Input: part model. Units: mm. Frame: model coordinates. Face numbers are marked on the shaded views. Coordinates: 2 decimals unless noted, no trailing zeros. Write each loop counter-clockwise with the first axis right and the second up, starting at its lowest first coordinate (ties: lowest second). Pieces come first, ordered by that corner, then holes.
1) Section query D-D (x = 15.5). Output: boundary loops of the cut face in (y, z).
2) Section query C-C (y = 4). State how many separate pieces and enclosed holes the cut face has, then the cut area to 3 significant figures.
3) Draft query along Y for the marked faces 1 and 2. Return one class per face: pulls with the +Y half, pulls with the -Y half, needs draft (parallel to the pull), parting line crosses it, or undercut.
4) Section query A-A (x = -4.85). Output: boundary loops of the cut face in (y, z), then the cut area to 4 significant figures.
5) Section query B-B (z = -15.5). Output: boundary loops of the cut face in (x, y), then the cut area to 4 significant figures.
6) Pin query (flat end, axial travel): pin 1 Ø4.5 at (x, z) = (15.15, -28.65) entering from -Y; pin 2 Ø3.5 at (x, z) = (-15.5, 15.5) entering from +Y. Return the tip coordinate at first contact, or that it passes through.
7) Line query: L1, parallel to Z at x = -15.5, y = 2.8; L2, parallel to X at y = 2.55, z = 28.65; L3, parallel to X at y = 2, z = 15.5. Output: solid intervals per line, ascending.
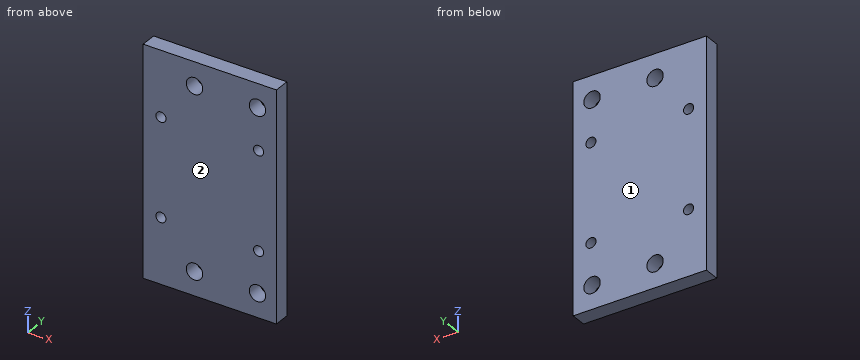
from build123d import *

# Parameters (mm, degrees)
SKETCH2_W           = 42.3
SKETCH2_H           = 42.3
SKETCH2_R           = 1.6
SKETCH2_H_2         = 15
SKETCH2_R_2         = 2.6
BOSS_EXTRUDE1_DEPTH = 5


with BuildPart() as part:
    # Sketch2 → Boss-Extrude1 (new body)
    with BuildSketch(Plane(origin=(0, 0, 0), x_dir=(1, 0, 0), z_dir=(0, 1, 0))):
        Rectangle(SKETCH2_W, SKETCH2_H)
        with Locations((-15.5, -15.5)):
            Circle(SKETCH2_R, mode=Mode.SUBTRACT)
        with Locations((15.5, 15.5)):
            Circle(SKETCH2_R, mode=Mode.SUBTRACT)
        with Locations((15.5, -15.5)):
            Circle(SKETCH2_R, mode=Mode.SUBTRACT)
        with Locations((-15.5, 15.5)):
            Circle(SKETCH2_R, mode=Mode.SUBTRACT)
        with Locations((0, -28.65)):
            Rectangle(SKETCH2_W, SKETCH2_H_2)
        with Locations((15.15, -28.65)):
            Circle(SKETCH2_R_2, mode=Mode.SUBTRACT)
        with Locations((-4.85, -28.65)):
            Circle(SKETCH2_R_2, mode=Mode.SUBTRACT)
        with Locations((0, 28.65)):
            Rectangle(SKETCH2_W, SKETCH2_H_2)
        with Locations((15.15, 28.65)):
            Circle(SKETCH2_R_2, mode=Mode.SUBTRACT)
        with Locations((-4.85, 28.65)):
            Circle(SKETCH2_R_2, mode=Mode.SUBTRACT)
    extrude(amount=BOSS_EXTRUDE1_DEPTH)


solid = part.part
Answer:
1. outline: (0, -36.15) - (5, -36.15) - (5, -31.23) - (0, -31.23) - close; (0, -26.07) - (5, -26.07) - (5, -17.1) - (0, -17.1) - close; (0, -13.9) - (5, -13.9) - (5, 13.9) - (0, 13.9) - close; (0, 17.1) - (5, 17.1) - (5, 26.07) - (0, 26.07) - close; (0, 31.23) - (5, 31.23) - (5, 36.15) - (0, 36.15) - close
2. separate pieces: 1
2. enclosed holes: 8
2. area: 2,940 mm2
3. face 1: pulls with the +Y half
3. face 2: pulls with the -Y half
4. outline: (0, -36.15) - (5, -36.15) - (5, -31.25) - (0, -31.25) - close; (0, -26.05) - (5, -26.05) - (5, 26.05) - (0, 26.05) - close; (0, 31.25) - (5, 31.25) - (5, 36.15) - (0, 36.15) - close
4. area: 309.5 mm2
5. outline: (-21.15, 0) - (-17.1, 0) - (-17.1, 5) - (-21.15, 5) - close; (-13.9, 0) - (13.9, 0) - (13.9, 5) - (-13.9, 5) - close; (17.1, 0) - (21.15, 0) - (21.15, 5) - (17.1, 5) - close
5. area: 179.5 mm2
6. pin 1: passes through
6. pin 2: stops at y = 5
7. L1: z = -36.15 to -17.1, -13.9 to 13.9, 17.1 to 36.15
7. L2: x = -21.15 to -7.45, -2.25 to 12.55, 17.75 to 21.15
7. L3: x = -21.15 to -17.1, -13.9 to 13.9, 17.1 to 21.15
